```python
from build123d import *

# Parameters (mm, degrees)
SKETCH_1_W          = 10
SKETCH_1_H          = 12
EXTRUDE_1_DEPTH     = 8
SKETCH_5_R          = 1
EXTRUDE_4_DEPTH     = 5
SKETCH_6_R          = 1
CUT_EXTRUDE_1_DEPTH = 16


with BuildPart() as part:
    # 草图1 → 凸台-拉伸1 (new body)
    with BuildSketch(Plane.XY):
        Rectangle(SKETCH_1_W, SKETCH_1_H)
    extrude(amount=EXTRUDE_1_DEPTH)

    # 草图5 → 凸台-拉伸4 (add)
    with BuildSketch(Plane(origin=(5, 0, 0), x_dir=(0, 0, -1), z_dir=(1, 0, 0))):
        with Locations(Location((-4, 0, 0), (0, 0, 180))):
            Circle(SKETCH_5_R)
    extrude(amount=EXTRUDE_4_DEPTH)

    # 草图6 → 切除-拉伸1 (cut)
    with BuildSketch(Plane.XZ.offset(6)):
        with Locations(Location((0, 4, 0), (0, 0, 270))):
            Circle(SKETCH_6_R)
    extrude(amount=-CUT_EXTRUDE_1_DEPTH, mode=Mode.SUBTRACT)


solid = part.part
```
Build history of the part. All positions in model axes, mm. Give positions to 0.01 mm unless a question says otherwise; leave off trailing zeros. Order: outer loops, then holes, each group sorted by start corner. A loop starts at its lowest first (then second) coordinate and runs counter-clockwise, first axis right, second up. Notation, with made-up numbers: M 29.25,18.5 L 77.25,18.5 A28 cw 77.25,40.5 Z; hole C 77,70.5 d11. An arc over 180 degrees is marked long. Write item = value, one per line. Start each with the question number.
(1) Slice it at B-B on z = 4. Write the cut outline in (x, y).
(2) Two-plate mould, pull along Z, no slides. Class faces 1 (the cylindrical face through (-0.6, -0.1, 4.8)), 2 (the cylindrical face through (7, 0, 3)), 3 (the flat face through (-1.2, 6, 3.9)): released by +Z, released by -Z, zero draft, split by the parting line, or undercut.
(3) Probe L1, parallel to X at y = -0.25, z = 4; L2, parallel to X at y = 3.25, z = 4; L3, parallel to X at y = -1, z = 1.75. List the from-to ranges inside material, lowest first. Write a range as [from, to].
(4) Slice it at A-A on x = 0. Write the cut outline in (y, z), plus the area to 3 significant figures.
(5) Slice it at D-D on y = 0. Write the cut outline in (x, z), plus the area to 3 significant figures.
(6) Pin check, flat tip, straight feed: pin 1 Ø3 at (y, z) = (4, 6) entering from +X. Stop position of the tip, or through.
(7) Slice it at C-C on y = -3.25. Write the cut outline in (x, z), plus the area to 3 significant figures.
Responses:
q1.outline = M -5,-6 L -1,-6 L -1,6 L -5,6 Z; M 1,-6 L 5,-6 L 5,-1 L 10,-1 L 10,1 L 5,1 L 5,6 L 1,6 Z
q2.face_1 = undercut
q2.face_2 = split by the parting line
q2.face_3 = zero draft
q3.L1 = [-5, -1], [1, 10]
q3.L2 = [-5, -1], [1, 5]
q3.L3 = [-5, 5]
q4.outline = M -6,0 L 6,0 L 6,3 L -6,3 Z; M -6,5 L 6,5 L 6,8 L -6,8 Z
q4.area = 72.0 mm2
q5.outline = M -5,0 L 5,0 L 5,3 L 10,3 L 10,5 L 5,5 L 5,8 L -5,8 Z; hole C 0,4 d2
q5.area = 86.9 mm2
q6.pin_1 = 5
q7.outline = M -5,0 L 5,0 L 5,8 L -5,8 Z; hole C 0,4 d2
q7.area = 76.9 mm2
